```python
from build123d import *

# Parameters (mm, degrees)
F0_W     = 92.291318
F0_H     = 56.53172
F1_DEPTH = 25
F2_T     = -1.5
F3_W     = 10
F3_H     = 10
F4_DEPTH = 8
F5_R     = 1.232119
F6_DEPTH = 6


with BuildPart() as f1:
    # F0 (on Top) → F1 (new body)
    with BuildSketch(Plane.XY):
        Rectangle(F0_W, F0_H)
    extrude(amount=F1_DEPTH)

    # F2
    f2_openings = [f1.faces().sort_by_distance(p)[0] for p in [
        (0, 0, 25),
    ]]
    offset(amount=F2_T, openings=f2_openings)

    # F3 (on face) → F4 (join)
    with BuildSketch(Plane.XY.offset(1.5)):
        with Locations((-39.645659, 21.76586)):
            Rectangle(F3_W, F3_H)
    extrude(amount=F4_DEPTH)

    # F5 (on face) → F6 (cut)
    with BuildSketch(Plane.XY.offset(9.5)):
        with Locations((-39.731406, 22.114344)):
            Circle(F5_R)
    extrude(amount=-F6_DEPTH, mode=Mode.SUBTRACT)


solid = f1.part
```
Source: CAD feature listing. Evaluate the final solid. Frame: model axes, mm. A direction names the side the tool comes from. Round coordinates to 2 decimals unless told otherwise and drop trailing zeros. Write each loop counter-clockwise with the first axis right and the second up, starting at its lowest first coordinate (ties: lowest second). Pieces come first, ordered by that corner, then holes. Notation, with made-up numbers: M 67.25,-9.75 L 98.25,-9.75 A22 cw 98.25,15.25 Z; hole C 6,8 d5. An arc over 180 degrees is marked long. Use CSV: the item, a comma, the result in double quotes. Start each with the question number.
Q1. Cut plane D-D on z = 7.5. Output: boundary loops of the cut face in (x, y), plus the area to 3 significant figures.
Q2. Cut plane C-C on x = -29. Output: boundary loops of the cut face in (y, z).
Q3. Line query: line 1 (X direction, y = 22, z = 15); line 2 (Y direction, x = 5.5, z = 19.75); line 3 (Z direction, x = 12.5, y = 20). Output: solid intervals per line, ascending. Write a range as from..to.
Q4. Access query for faces 1 (the face through (-1, -28.266, 12)), 2 (the face through (44.646, 0, 13)). Directions: +Z, -Z, +X, -X, +Y, -Y. A direction counts if a zero-diameter tool reaches every point of the face in a straight line with its end or side. Return the directions, or none.
Q5. Pull-direction query (X, two-part tool) for faces 3 (the face through (-14, -27, 25)), 4 (the face through (-34.646, 22, 5)), 5 (the face through (46.146, 0, 12)); classes: +X half, -X half, draft (parallel to the pull), parting line (faces both ways), or undercut.
Q6. Cut plane A-A on z = 11.5. Output: boundary loops of the cut face in (x, y), plus the area to 3 significant figures.
Q7. First-contact query: P1, Ø6, axis at x = -21.5, y = -13, coming from the +Z side; P2, Ø5, axis at x = -39.5, y = 22.5, coming from the +Z side. Flat tips, straight axial feed; report the tip coordinate or a pass-through.
Q8. Cut plane B-B on y = 4. Output: boundary loops of the cut face in (x, z).
Results found:
1,outline,"M -46.15,-28.27 L 46.15,-28.27 L 46.15,28.27 L -46.15,28.27 Z; hole M -44.65,-26.77 L 44.65,-26.77 L 44.65,26.77 L -34.65,26.77 L -34.65,16.77 L -44.65,16.77 Z; hole C -39.73,22.11 d2.46"
1,area,"533 mm^2"
2,outline,"M -28.27,0 L 28.27,0 L 28.27,25 L 26.77,25 L 26.77,1.5 L -26.77,1.5 L -26.77,25 L -28.27,25 Z"
3,line 1,"-46.15..-44.65, 44.65..46.15"
3,line 2,"-28.27..-26.77, 26.77..28.27"
3,line 3,"0..1.5"
4,face 1,"+Z, -Z, +X, -X, -Y"
4,face 2,"+Z"
5,face 3,"draft"
5,face 4,"undercut"
5,face 5,"+X half"
6,outline,"M -46.15,-28.27 L 46.15,-28.27 L 46.15,28.27 L -46.15,28.27 Z; hole M -44.65,-26.77 L 44.65,-26.77 L 44.65,26.77 L -44.65,26.77 Z"
6,area,"437 mm^2"
7,P1,"z = 1.5"
7,P2,"z = 9.5"
8,outline,"M -46.15,0 L 46.15,0 L 46.15,25 L 44.65,25 L 44.65,1.5 L -44.65,1.5 L -44.65,25 L -46.15,25 Z"
